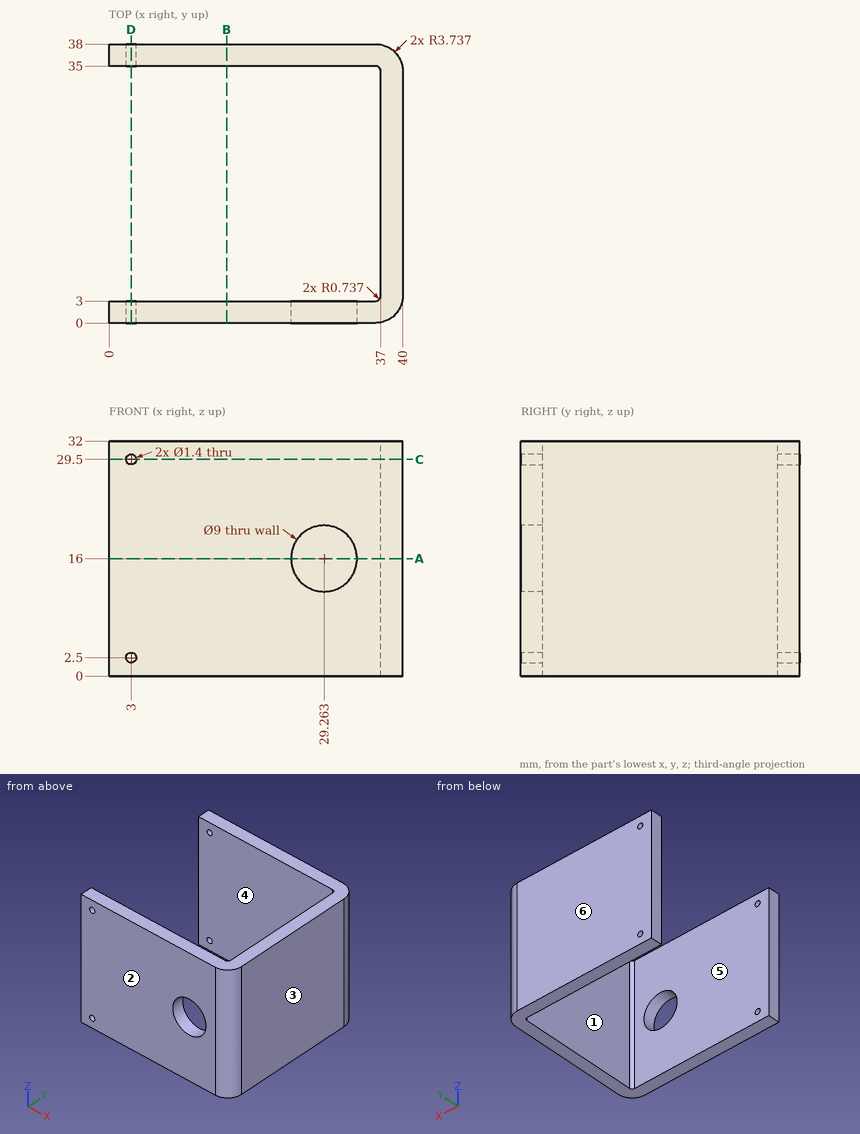
The figure shows three views and two pictorial views of one solid part (mm, origin at its lowest corner). Answer the questions. A direction names the side the tool comes from. Round coordinates to 2 decimals unless told otherwise and drop trailing zeros. Order: outer loops, then holes, each group sorted by start corner. A loop starts at its lowest first (then second) coordinate and runs counter-clockwise, first axis right, second up.
Q1. A cutting plane is placed at D-D, the plane x = 3. Determine the outline of the cut face in (y, z), then the cut area to 3 significant figures.
Solution:
outline: (0, 0) - (3, 0) - (3, 1.8) - (0, 1.8) - close; (0, 3.2) - (3, 3.2) - (3, 28.8) - (0, 28.8) - close; (0, 30.2) - (3, 30.2) - (3, 32) - (0, 32) - close; (35, 0) - (38, 0) - (38, 1.8) - (35, 1.8) - close; (35, 3.2) - (38, 3.2) - (38, 28.8) - (35, 28.8) - close; (35, 30.2) - (38, 30.2) - (38, 32) - (35, 32) - close
area: 175 mm2
Q2. A cutting plane is placed at A-A, the plane z = 16. Determine the outline of the cut face in (x, y).
Solution:
outline: (0, 0) - (24.76, 0) - (24.76, 3) - (0, 3) - close; (0, 35) - (36.26, 35) arc R0.74 cw to (37, 34.26) - (37, 3.74) arc R0.74 cw to (36.26, 3) - (33.76, 3) - (33.76, 0) - (36.26, 0) arc R3.74 ccw to (40, 3.74) - (40, 34.26) arc R3.74 ccw to (36.26, 38) - (0, 38) - close
Q3. A tool of negligible diameter and unlimited length cuts with its end or side. For the marked faces 5 and 6, from which of +Z, -Z, +X, -X, +Y, -Y can it reach the whole face along a straight path? Write none if from no direction.
Solution:
face 5: +Z, -Z, -X
face 6: +Z, -Z, +X, -X, +Y
Q4. Given pin 1 Ø5.5 at (x, z) = (29.26, 16) entering from -Y; pin 2 Ø9 at (y, z) = (15, 12) entering from -X; pin 3 Ø0.8 at (x, z) = (3, 29.5) entering from +Y, each flat-ended and moving along its own axis, determine where each tip first touches the part or whether it passes through.
Solution:
pin 1: stops at y = 35
pin 2: stops at x = 37
pin 3: passes through
Q5. A cutting plane is placed at C-C, the plane z = 29.5. Determine the outline of the cut face in (x, y).
Solution:
outline: (0, 0) - (2.3, 0) - (2.3, 3) - (0, 3) - close; (0, 35) - (2.3, 35) - (2.3, 38) - (0, 38) - close; (3.7, 0) - (36.26, 0) arc R3.74 ccw to (40, 3.74) - (40, 34.26) arc R3.74 ccw to (36.26, 38) - (3.7, 38) - (3.7, 35) - (36.26, 35) arc R0.74 cw to (37, 34.26) - (37, 3.74) arc R0.74 cw to (36.26, 3) - (3.7, 3) - close
Q6. Find the intervals of material crossed by line 1 along Y through (x, z) = (33.5, 21); line 2 along X through (y, z) = (25.5, 29); line 3 along Y through (x, z) = (31, 17.5), in increasing order.
Solution:
line 1: y = 0 to 3, 35 to 38
line 2: x = 37 to 40
line 3: y = 35 to 38
Q7. The mould has two halves that part along Y. Classify the marked faces 1, 2, 3 and 4: pulls with the +Y half, pulls with the -Y half, needs draft (parallel to the pull), parting line crosses it, or undercut.
Solution:
face 1: undercut
face 2: pulls with the -Y half
face 3: needs draft
face 4: undercut
Q8. A cutting plane is placed at B-B, the plane x = 16. Determine the outline of the cut face in (y, z).
Solution:
outline: (0, 0) - (3, 0) - (3, 32) - (0, 32) - close; (35, 0) - (38, 0) - (38, 32) - (35, 32) - close
